```python
from build123d import *

# Parameters (mm, degrees)
PAD006_DEPTH           = 65
POCKET_DEPTH           = 63
SKETCH009_R            = 16.1
POCKET005_DEPTH        = 346.001
PAD009_DEPTH           = 10
LINEARPATTERN_COUNT    = 2
LINEARPATTERN_PITCH    = 103
LINEARPATTERN001_COUNT = 2
LINEARPATTERN001_PITCH = 103
SKETCH016_W            = 3
SKETCH016_H            = 5
PAD010_DEPTH           = 75
SKETCH020_W            = 10
SKETCH020_H            = 5
PAD011_DEPTH           = 6
CHAMFER001_SIZE        = 1.9
SKETCH021_W            = 7
SKETCH021_H            = 7
POCKET007_DEPTH        = 1.5
LINEARPATTERN002_COUNT = 2
LINEARPATTERN002_PITCH = 103
LINEARPATTERN003_COUNT = 2
LINEARPATTERN003_PITCH = 103
CHAMFER003_SIZE        = 2.2
CHAMFER008_SIZE        = 3.9


with BuildPart() as part:
    # Sketch007 → Pad006 (new body)
    with BuildSketch(Plane.XY):
        with BuildLine():
            Line((-173, 20), (-173, -20))
            ThreePointArc((-173, -20), (-170.071068, -27.071068), (-163, -30))
            Line((-163, -30), (163, -30))
            ThreePointArc((163, -30), (170.071068, -27.071068), (173, -20))
            Line((173, -20), (173, 20))
            ThreePointArc((173, 20), (170.071068, 27.071068), (163, 30))
            Line((163, 30), (-163, 30))
            ThreePointArc((-163, 30), (-170.071068, 27.071068), (-173, 20))
        make_face()
    extrude(amount=PAD006_DEPTH)

    # Sketch008 → Pocket (cut)
    with BuildSketch(Plane.XY):
        with BuildLine():
            Line((-170, 18), (-170, -18))
            ThreePointArc((-170, -18), (-167.071068, -25.071068), (-160, -28))
            Line((-160, -28), (160, -28))
            ThreePointArc((160, -28), (167.071068, -25.071068), (170, -18))
            Line((170, -18), (170, 18))
            ThreePointArc((170, 18), (167.071068, 25.071068), (160, 28))
            Line((160, 28), (-160, 28))
            ThreePointArc((-160, 28), (-167.071068, 25.071068), (-170, 18))
        make_face()
    extrude(amount=POCKET_DEPTH, mode=Mode.SUBTRACT)

    # Sketch009 → Pocket005 (cut, through all)
    with BuildSketch(Plane(origin=(-173, 0, 0), x_dir=(0, -1, 0), z_dir=(-1, 0, 0))):
        with Locations((0, 35)):
            Circle(SKETCH009_R)
    extrude(amount=-POCKET005_DEPTH, mode=Mode.SUBTRACT)

    # Sketch017 → Pad009 (join, symmetric)
    with BuildSketch(Plane.YZ):
        Polygon((-28, 63), (28, 63), (28, 10), (26, 20), (26, 59), (-26, 59), (-26, 15), (-28, 2.2), align=None)
    pad009 = extrude(amount=PAD009_DEPTH, both=True)

    # LinearPattern: Pad009 ×2
    with Locations(*[(-i * LINEARPATTERN_PITCH, 0, 0) for i in range(1, LINEARPATTERN_COUNT)]):
        add(pad009)

    # LinearPattern001: Pad009 ×2
    with Locations(*[(i * LINEARPATTERN001_PITCH, 0, 0) for i in range(1, LINEARPATTERN001_COUNT)]):
        add(pad009)

    # Sketch016 → Pad010 (join, symmetric)
    with BuildSketch(Plane.YZ):
        with Locations((-26.5, 4.7)):
            Rectangle(SKETCH016_W, SKETCH016_H)
    extrude(amount=PAD010_DEPTH, both=True)

    # Sketch020 (on Face1 of Pad010) → Pad011 (join)
    with BuildSketch(Plane(origin=(-173, 0, 0), x_dir=(0, -1, 0), z_dir=(-1, 0, 0))):
        with Locations((0, 60.5)):
            Rectangle(SKETCH020_W, SKETCH020_H)
    extrude(amount=-PAD011_DEPTH)

    # Chamfer001
    chamfer001_edges = [part.edges().sort_by_distance(p)[0] for p in [
        (113, -26, 37),
        (113, 26, 39.5),
        (10, 26, 39.5),
        (10, -26, 37),
        (-93, -26, 37),
        (-93, 26, 39.5),
        (-113, 26, 39.5),
        (-113, -26, 37),
        (-10, -26, 37),
        (-10, 26, 39.5),
        (93, 26, 39.5),
        (93, -26, 37),
    ]]
    chamfer(chamfer001_edges, length=CHAMFER001_SIZE)

    # Sketch021 → Pocket007 (cut)
    with BuildSketch(Plane.XY.offset(65)):
        Rectangle(SKETCH021_W, SKETCH021_H)
    pocket007 = extrude(amount=-POCKET007_DEPTH, mode=Mode.SUBTRACT)

    # LinearPattern002: Pocket007 ×2
    with Locations(*[(i * LINEARPATTERN002_PITCH, 0, 0) for i in range(1, LINEARPATTERN002_COUNT)]):
        add(pocket007, mode=Mode.SUBTRACT)

    # LinearPattern003: Pocket007 ×2
    with Locations(*[(-i * LINEARPATTERN003_PITCH, 0, 0) for i in range(1, LINEARPATTERN003_COUNT)]):
        add(pocket007, mode=Mode.SUBTRACT)

    # Chamfer003
    chamfer003_edges = [part.edges().sort_by_distance(p)[0] for p in [
        (75, -25, 4.7),
        (0, -25, 7.2),
        (-75, -25, 4.7),
    ]]
    chamfer(chamfer003_edges, length=CHAMFER003_SIZE)

    # Chamfer008
    chamfer008_edges = [part.edges().sort_by_distance(p)[0] for p in [
        (113, 0, 59),
        (93, 0, 59),
        (10, 0, 59),
        (-10, 0, 59),
        (-93, 0, 59),
        (-113, 0, 59),
    ]]
    chamfer(chamfer008_edges, length=CHAMFER008_SIZE)


with BuildPart() as part_1:
    # Body002 placement: moved
    add(part.part.moved(Location((0, 0, -60))))


solid = part_1.part
```
Verification items for the finished model (mm, model axes). A direction names the side the tool comes from. Give positions to 0.01 mm unless a question says otherwise; leave off trailing zeros. Order: outer loops, then holes, each group sorted by start corner. A loop starts at its lowest first (then second) coordinate and runs counter-clockwise, first axis right, second up. Notation, with made-up numbers: M 53.25,-10 L 62.25,-10 A20 cw 62.25,24 Z; hole C 26,69.5 d10. An arc over 180 degrees is marked long. Return JSON: item names as keys, results as strings. Group by question number.
1) Section check A-A on x = -32.5. Record the cut outline in (y, z), and give its area (3 significant figures).
2) Go/stop test with flat-tipped pins: pin 1 Ø2.5 at (x, z) = (-168.5, 1) entering from +Y; pin 2 Ø5 at (y, z) = (-24, -14.5) entering from -X; pin 3 Ø3 at (x, y) = (8.5, 17.5) entering from -Z. Record where each tip stops, or that it passes through.
3) Mould release check, pull along X, two halves, no side actions. Record for faces 1 (the face through (170.15, 26.99, -27.96)), 2 (the face through (171.479, -15.357, -20.164)), 3 (the face through (0, 27, -45)): pulls with the +X half, pulls with the -X half, needs draft (parallel to the pull), parting line crosses it, or undercut.
4) Section check B-B on y = 8.5. Give the number of separate pieces and of enclosed holes in the cut face, and give its area (3 significant figures).
5) Scan lines: line 1 (Y direction, x = 78, z = -41.5); line 2 (Z direction, x = 172, y = 0); line 3 (X direction, y = 5, z = -52). Record each from-to range of solid material in increasing order.
6) Access from +Z, -Z, +X, -X, +Y, -Y to the whole of each face (thin tool, end or side, straight path). Record for faces 4 (the face through (-167.15, -24.99, -28.94)), 5 (the face through (-171.521, -15.357, -20.164)), 6 (the face through (0, -26, -22)).
Answer block:
{
 "1": {"outline": "M -30,-60 L -28,-60 L -28,-57.8 L -25,-57.8 L -25,-55 L -27.2,-52.8 L -28,-52.8 L -28,3 L 28,3 L 28,-60 L 30,-60 L 30,5 L -30,5 Z", "area": "385 mm^2"},
 "2": {"pin 1": "stops at y = 29.05", "pin 2": "stops at x = -172.89", "pin 3": "stops at z = -0.1"},
 "3": {"face 1": "pulls with the +X half", "face 2": "needs draft", "face 3": "undercut"},
 "4": {"separate pieces": "3", "enclosed holes": "0", "area": "1,100 mm^2"},
 "5": {"line 1": "y = -30 to -28, 28 to 30", "line 2": "z = -60 to -41.1, -8.9 to 5", "line 3": "x = -173 to -170, 170 to 173"},
 "6": {"face 4": "-Z", "face 5": "+X, -X", "face 6": "none"}
}
